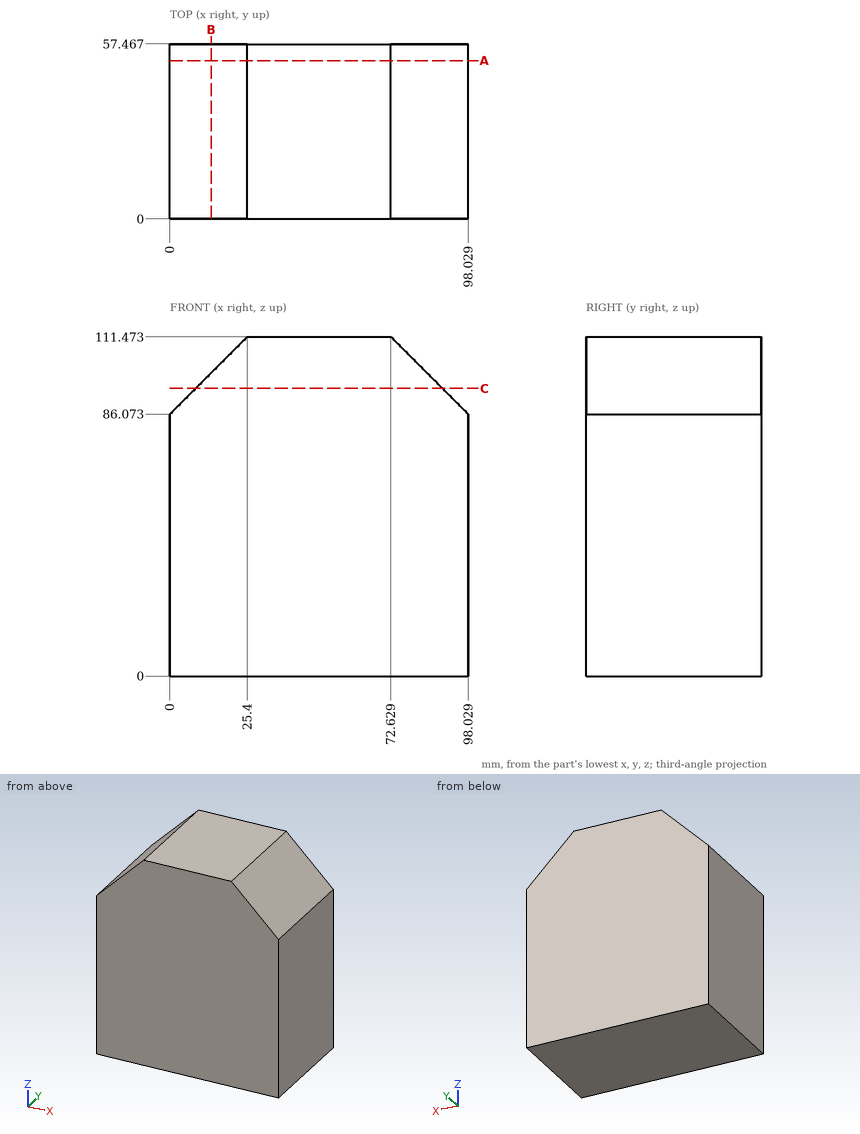
Geometry: see drawing. Coordinates: mm, zero at the bounding-box minimum. Give positions to 0.01 mm unless a question says otherwise; leave off trailing zeros. Loops run counter-clockwise (first coordinate to the right, second up) from the corner with the lowest first, then second, coordinate; pieces in that order, holes last. Notation, with made-up numbers: M 17.25,-19 L 30.25,-19 A31 ccw 30.25,19 Z; hole C 73,31.25 d1. An arc over 180 degrees is marked long. Answer as CSV lines item,"result". Start each with the question number.
1. Section C-C on z = 94.5. Return loops of the section in (x, y), plus the area to 4 significant figures.
2. Section A-A on y = 52. Return loops of the section in (x, z), plus the area to 3 significant figures.
3. Line query: L1, parallel to Z at x = 14, y = 5.5 (1 decimal); L2, parallel to Z at x = 89.5, y = 54; L3, parallel to X at y = 38.5, z = 97 (1 decimal). Output: solid intervals per line, ascending.
4. Section B-B on x = 13.5. Return loops of the section in (y, z).
Computed values:
1,outline,"M 8.43,0 L 89.6,0 L 89.6,57.47 L 8.43,57.47 Z"
1,area,"4,665 mm²"
2,outline,"M 0,0 L 98.03,0 L 98.03,86.07 L 72.63,111.47 L 25.4,111.47 L 0,86.07 Z"
2,area,"10,300 mm²"
3,L1,"z = 0 to 100.1"
3,L2,"z = 0 to 94.6"
3,L3,"x = 10.9 to 87.1"
4,outline,"M 0,0 L 57.47,0 L 57.47,99.57 L 0,99.57 Z"
